from build123d import *

# Parameters (mm, degrees)
F2_SIZE = 0.75
F3_SIZE = 0.1


with BuildPart() as f1:
    # F0 (on Front) → F1 (revolve)
    with BuildSketch(Plane.XZ):
        Polygon((-11, 2.6), (-11, 0), (-3.97, 0), (-3.97, -3.5), (-2.663974, -3.5), (-2.663974, 2.6), align=None)
    revolve(axis=Axis((0, 0, -0.45), (0, 0, -1)))

    # F2
    f2_edges = [f1.edges().sort_by_distance(p)[0] for p in [
        (11, 0, 2.6),
    ]]
    chamfer(f2_edges, length=F2_SIZE)

    # F3
    f3_edges = [f1.edges().sort_by_distance(p)[0] for p in [
        (2.663974, 0, 2.6),
    ]]
    chamfer(f3_edges, length=F3_SIZE)


solid = f1.part
The model under review builds one solid part; all positions refer to its coordinate system, in mm. A direction names the side the tool comes from. Give positions to 0.01 mm unless a question says otherwise; leave off trailing zeros. Order: outer loops, then holes, each group sorted by start corner. A loop starts at its lowest first (then second) coordinate and runs counter-clockwise, first axis right, second up. Notation, with made-up numbers: M 47,-39.75 L 61,-39.75 A11 cw 61,-21.75 Z; hole C -37,-40 d3. An arc over 180 degrees is marked long. One line per question, with ' | ' between items. Start each with the question number.
1) Consider section C-C, the plane z = 1. Give the boundary of the cut face in (x, y), then the cut area to 3 significant figures.
2) Consider section A-A, the plane y = 0. Give the boundary of the cut face in (x, z), then the cut area to 3 significant figures.
3) For faces 1 (the face through (-3.787, 1.192, -1.774)), 2 (the face through (2.114, -1.621, -0.458)), list the 3-axis set-ups (+Z, -Z, +X, -X, +Y, -Y) from which the entire face can be reached by the end or side of a thin tool; tool diameter is ignored.
4) Clearance check with flat-ended pins moving along their axes: P1, Ø1.5, axis at y = 2, z = 1.5, coming from the +X side; P2, Ø2, axis at y = -2, z = -2, coming from the -X side; P3, Ø3, axis at x = -6.5, z = 1, coming from the +Y side. State where each tip first meets the part, or that it passes through.
5) Wall thickness on L1, parallel to Y at x = 0, z = -0.9; L2, parallel to Y at x = 0, z = 0.6; L3, parallel to Z at x = 5, y = 3: over which ranges is each line inside the solid? List them lowest first. Write a range as from..to.
6) Consider section D-D, the plane z = -1.75. Give the boundary of the cut face in (x, y).
Found:
1) outline: C 0,0 d22; hole C 0,0 d5.33 | area: 358 mm²
2) outline: M -11,0 L -3.97,0 L -3.97,-3.5 L -2.66,-3.5 L -2.66,2.5 L -2.76,2.6 L -10.25,2.6 L -11,1.85 Z; M 2.66,-3.5 L 3.97,-3.5 L 3.97,0 L 11,0 L 11,1.85 L 10.25,2.6 L 2.76,2.6 L 2.66,2.5 Z | area: 51.9 mm²
3) face 1: -Z | face 2: +Z, -Z
4) P1: stops at x = 10.93 | P2: stops at x = -3.84 | P3: stops at y = 9.8
5) L1: y = -3.97..-2.66, 2.66..3.97 | L2: y = -11..-2.66, 2.66..11 | L3: z = 0..2.6
6) outline: C 0,0 d7.94; hole C 0,0 d5.33
